The drawing under review shows one solid part. Ordinate dimensions are in mm from its lowest x, y, z. Coordinates: 2 decimals unless noted, no trailing zeros. Order: outer loops, then holes, each group sorted by start corner. A loop starts at its lowest first (then second) coordinate and runs counter-clockwise, first axis right, second up. Notation, with made-up numbers: (34.25, -7) -> (92.25, -7) arc R21 cw to (92.25, 30) -> close; hole circle Ø10 at (69, 7). An arc over 180 degrees is marked (long way). Put each result on its own line as item: value.
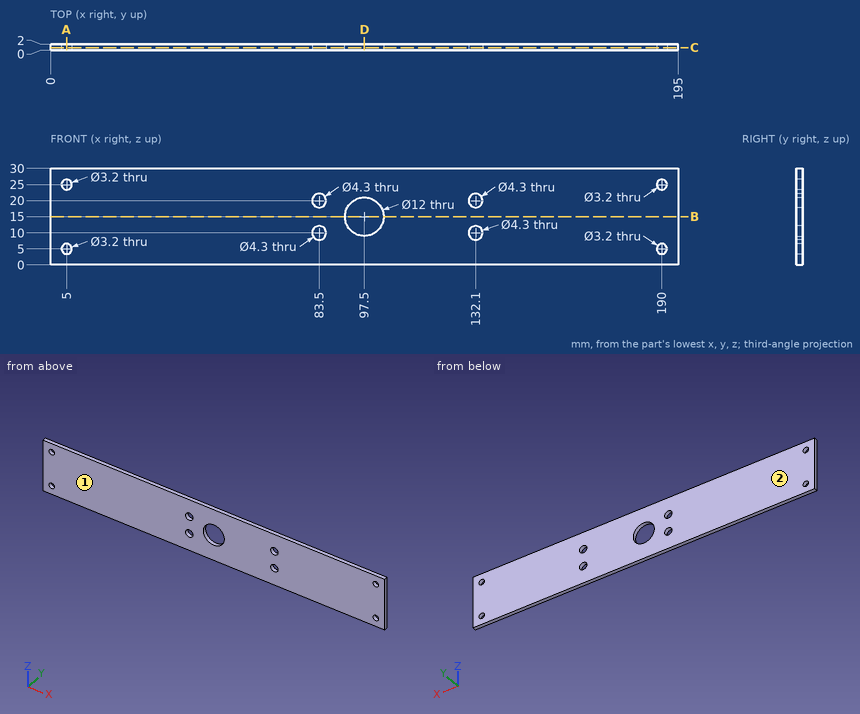
Item 1: Consider section C-C on y = 0.85. Count the separate pieces of the cut face and the enclosed holes in it, and give its area (3 significant figures).
Answers below:
separate pieces: 1
enclosed holes: 9
area: 5,650 mm^2
Item 2: Consider section A-A on x = 5. Write out the cut boundary in (y, z), and give its area (3 significant figures).
Answers below:
outline: (0, 0) -> (2, 0) -> (2, 3.4) -> (0, 3.4) -> close; (0, 6.6) -> (2, 6.6) -> (2, 23.4) -> (0, 23.4) -> close; (0, 26.6) -> (2, 26.6) -> (2, 30) -> (0, 30) -> close
area: 47.2 mm^2
Item 3: Mouldability with a two-part tool opening along Y and no side actions: class the marked faces 1 and 2 as +Y half, -Y half, draft (parallel to the pull), parting line (faces both ways), or undercut.
Answers below:
face 1: -Y half
face 2: +Y half
Item 4: For line 1 (Z direction, x = 5, y = 0.55); line 2 (X direction, y = 1.4, z = 5); line 3 (Z direction, x = 132.1, y = 0.45), list the stretches that pass through material, from the lowest coordinate up. Write a range as from..to.
Answers below:
line 1: 0..3.4, 6.6..23.4, 26.6..30
line 2: 0..3.4, 6.6..188.4, 191.6..195
line 3: 0..7.85, 12.15..17.85, 22.15..30
Item 5: For pin 1 Ø2.5 at (x, z) = (5, 5) entering from +Y, flat-tipped, find the tip position at first contact; note if it passes through.
Answers below:
pin 1: through
Item 6: Consider section B-B on z = 15. Write out the cut boundary in (x, y), and give its area (3 significant figures).
Answers below:
outline: (0, 0) -> (91.5, 0) -> (91.5, 2) -> (0, 2) -> close; (103.5, 0) -> (195, 0) -> (195, 2) -> (103.5, 2) -> close
area: 366 mm^2
Item 7: Consider section D-D on x = 97.5. Write out the cut boundary in (y, z).
Answers below:
outline: (0, 0) -> (2, 0) -> (2, 9) -> (0, 9) -> close; (0, 21) -> (2, 21) -> (2, 30) -> (0, 30) -> close
